Geometry: final body of the model. Coordinates: model frame, mm. A direction names the side the tool comes from. Round coordinates to 2 decimals unless told otherwise and drop trailing zeros. Loops run counter-clockwise (first coordinate to the right, second up) from the corner with the lowest first, then second, coordinate; pieces in that order, holes last. Notation, with made-up numbers: (-18, 11.5) - (38, 11.5) arc R18 ccw to (38, 41.5) - close; hole circle Ø4 at (21.25, 68). An arc over 180 degrees is marked (long way). Answer as CSV lines item,"result".
from build123d import *

# Parameters (mm, degrees)
BOSS_EXTRUDE1_DEPTH = 29
SKETCH2_W           = 1
SKETCH2_H           = 24.95
BOSS_EXTRUDE2_DEPTH = 100
SKETCH4_W           = 1
SKETCH4_H           = 24.95
BOSS_EXTRUDE3_DEPTH = 101.96257304
CUT_EXTRUDE1_DEPTH  = 1
SKETCH6_R           = 0.498897706
CUT_EXTRUDE2_DEPTH  = 1
FILLET1_R           = 2


with BuildPart() as part:
    # Sketch1 → Boss-Extrude1 (new body)
    with BuildSketch(Plane(origin=(0, 0, 0), x_dir=(1, 0, 0), z_dir=(0, 1, 0))):
        Polygon((-20.5, 0), (20.5, 0), (41.08, -4), (47.08, -4), (67, -4), (67, -1.96257304), (47.08, -1.96257304), (41.08, -1.96257304), (20.69256171, 2), (-20.5, 2), align=None)
    extrude(amount=BOSS_EXTRUDE1_DEPTH)

    # Sketch2 → Boss-Extrude2 (add)
    with BuildSketch(Plane(origin=(0, 0, 1.96257304), x_dir=(-1, 0, 0), z_dir=(0, 0, -1))):
        with Locations((-64.5, 14.5)):
            Rectangle(SKETCH2_W, SKETCH2_H)
    extrude(amount=-BOSS_EXTRUDE2_DEPTH)

    # Sketch4 → Boss-Extrude3 (add)
    with BuildSketch(Plane.XY):
        with Locations((-18, 14.5)):
            Rectangle(SKETCH4_W, SKETCH4_H)
    extrude(amount=BOSS_EXTRUDE3_DEPTH)

    # Sketch5 → Cut-Extrude1 (cut)
    with BuildSketch(Plane.ZY.offset(18.5)):
        with BuildLine():
            Line((1.95, 19.17), (2.66, 19.17))
            ThreePointArc((2.66, 19.17), (3.685304833, 18.745304833), (4.11, 17.72))
            Line((4.11, 17.72), (4.11, 11.28))
            ThreePointArc((4.11, 11.28), (3.685304833, 10.254695167), (2.66, 9.83))
            Line((2.66, 9.83), (1.95, 9.83))
            ThreePointArc((1.95, 9.83), (0.924695167, 10.254695167), (0.5, 11.28))
            Line((0.5, 11.28), (0.5, 17.72))
            ThreePointArc((0.5, 17.72), (0.924695167, 18.745304833), (1.95, 19.17))
        make_face()
    extrude(amount=-CUT_EXTRUDE1_DEPTH, mode=Mode.SUBTRACT)

    # Sketch6 → Cut-Extrude2 (cut)
    with BuildSketch(Plane.ZY.offset(18.5)):
        with Locations(Location((4.61, 8.645, 0), (0, 0, 270))):
            Circle(SKETCH6_R)
    extrude(amount=-CUT_EXTRUDE2_DEPTH, mode=Mode.SUBTRACT)

    # Fillet1
    fillet1_edges = [part.edges().sort_by_distance(p)[0] for p in [
        (0.096280855, 0, -2),
        (30.886280855, 0, -0.01871348),
        (54.04, 0, 1.96257304),
        (67, 0, 2.98128652),
        (-20.5, 0, -1),
        (-20.5, 14.5, -2),
        (20.69256171, 14.5, -2),
        (41.08, 14.5, 1.96257304),
        (67, 14.5, 1.96257304),
        (67, 29, 2.98128652),
        (54.04, 29, 1.96257304),
        (30.886280855, 29, -0.01871348),
        (0.096280855, 29, -2),
        (-20.5, 29, -1),
    ]]
    fillet(fillet1_edges, radius=FILLET1_R - 0.0001)  # a hair under: the kernel refuses the full size


solid = part.part
(1) Access query for faces 1 (the face through (30.646, 14.297, 1.972)), 2 (the face through (65, 14, 52)), 3 (the face through (30.637, 28.399, 0.514)), 4 (the face through (53, 15, 1.963)), 5 (the face through (-18.5, 14, 50)). Directions: +Z, -Z, +X, -X, +Y, -Y. A direction counts if a zero-diameter tool reaches every point of the face in a straight line with its end or side. Return the directions, or none.
Findings below:
face 1,"+Z, +Y, -Y"
face 2,"+Z, +X, +Y, -Y"
face 3,"-Z, +X, +Y"
face 4,"-Z, +X, +Y, -Y"
face 5,"+Z, -X, +Y, -Y"
(2) Pin query (flat end, axial travel): P1, Ø3, axis at y = 26, z = 27.5, coming from the +X side; P2, Ø1.1, axis at x = 64.5, z = 36, coming from the +Y side (3 decimals); P3, Ø1.5, axis at x = 36.5, y = 5.5, coming from the -Z side. Return the tip coordinate at first contact, or that it passes through.
Findings below:
P1,"x = 65"
P2,"y = 26.975"
P3,"z = 0.93"
(3) Material intervals for line 1 along X through (y, z) = (12.75, 58.5); line 2 along Z through (x, y) = (13, 16); line 3 along Z through (x, y) = (52, 25), sorted ascending.
Findings below:
line 1,"-18.5 to -17.5, 64 to 65"
line 2,"-2 to 0"
line 3,"1.96 to 4"
(4) Section B-B (z = 12). Output: boundary loops of the cut face in (x, y) (3 decimals), and give its area (3 significant figures).
Findings below:
outline,"(-18.5, 2.025) - (-17.5, 2.025) - (-17.5, 26.975) - (-18.5, 26.975) - close; (64, 2.025) - (65, 2.025) - (65, 26.975) - (64, 26.975) - close"
area,"49.9 mm2"
(5) Draft query along X for faces 6 (the face through (64, 14, 52)), 7 (the face through (0, 14, 0)), 8 (the face through (30.631, 0.57, 0.544)), 9 (the face through (1, 14, -2)). Return one class per face: pulls with the +X half, pulls with the -X half, needs draft (parallel to the pull), parting line crosses it, or undercut.
Findings below:
face 6,"undercut"
face 7,"undercut"
face 8,"pulls with the +X half"
face 9,"needs draft"
